from build123d import *

# Parameters (mm, degrees)
SKETCH1_R           = 2
BOSS_EXTRUDE1_DEPTH = 1.4077243
FILLET2_R           = 4


with BuildPart() as part:
    # Sketch1 → Boss-Extrude1 (new body)
    with BuildSketch(Plane(origin=(0, 0, 0), x_dir=(1, 0, 0), z_dir=(0, 1, 0))):
        Polygon((6, -8), (6, 33.34843691), (-61.475760907, 128.370940703), (-81.524239093, 119.312324779), (-104.126855641, 18.58956294), (-104.126855641, -8), align=None)
        with Locations(Location((-96, 0, 0), (0, 0, 270))):
            Circle(SKETCH1_R, mode=Mode.SUBTRACT)
        with Locations(Location((-80, 0, 0), (0, 0, 270))):
            Circle(SKETCH1_R, mode=Mode.SUBTRACT)
        with Locations(Location((-64, 0, 0), (0, 0, 270))):
            Circle(SKETCH1_R, mode=Mode.SUBTRACT)
        with Locations(Location((-97.021679837, 31.983686003, 0), (0, 0, 270))):
            Circle(SKETCH1_R, mode=Mode.SUBTRACT)
        with Locations(Location((-48, 0, 0), (0, 0, 270))):
            Circle(SKETCH1_R, mode=Mode.SUBTRACT)
        with Locations(Location((-32, 0, 0), (0, 0, 270))):
            Circle(SKETCH1_R, mode=Mode.SUBTRACT)
        with Locations(Location((-16, 0, 0), (0, 0, 270))):
            Circle(SKETCH1_R, mode=Mode.SUBTRACT)
        with Locations(Location((0, 0, 0), (0, 0, 270))):
            Circle(SKETCH1_R, mode=Mode.SUBTRACT)
        with Locations(Location((-67.5, 116.913429511, 0), (0, 0, 270))):
            Circle(SKETCH1_R, mode=Mode.SUBTRACT)
    extrude(amount=BOSS_EXTRUDE1_DEPTH)

    # Fillet2
    fillet2_edges = [part.edges().sort_by_distance(p)[0] for p in [
        (6, 0.70386215, 8),
        (-104.126855641, 0.70386215, 8),
        (-104.126855641, 0.70386215, -18.58956294),
        (-81.524239093, 0.70386215, -119.312324779),
        (-61.475760907, 0.70386215, -128.370940703),
        (6, 0.70386215, -33.34843691),
    ]]
    fillet(fillet2_edges, radius=FILLET2_R)


solid = part.part
Check sheet for the modelled part. Datum: model origin and axes. Units: mm. Give positions to 0.01 mm unless a question says otherwise; leave off trailing zeros. Loops run counter-clockwise (first coordinate to the right, second up) from the corner with the lowest first, then second, coordinate; pieces in that order, holes last. Notation, with made-up numbers: M 80.25,13.5 L 125.25,13.5 A11 cw 125.25,32.5 Z; hole C 36,71 d10. An arc over 180 degrees is marked long. Return JSON: item names as keys, results as strings. Group by question number.
1. Mould release check, pull along Z, two halves, no side actions. Record for faces 1 (the flat face through (-71.985, 0.694, -123.623)), 2 (the cylindrical face through (-2, 1, 0)), 3 (the flat face through (-50, 0, -46)), 4 (the cylindrical face through (-102.924, 0.714, 6.859)): released by +Z, released by -Z, zero draft, split by the parting line, or undercut.
2. Cross-section at A-A on z = 0. State how many separate pieces and enclosed holes the cut face has, plus the area to 3 significant figures.
3. Thickness scan on L1, parallel to X at y = 0.5, z = -32.5; L2, parallel to Z at x = -48.5, y = 0.55; L3, parallel to X at y = 0.85, z = -53.5. Record the ranges inside material, lowest first.
4. Cross-section at B-B on x = -48. Record the boundary of the cut face in (y, z), plus the area to 3 significant figures.
5. Go/stop test with a flat-tipped pin: pin 1 (2.5 mm diameter, centred on x = -80, z = 0, fed in from +Y). Record where the tip stops, or that it passes through.
6. Cross-section at D-D on x = -16. Record the boundary of the cut face in (y, z), plus the area to 3 significant figures.
Return value:
{
 "1": {"face 1": "released by -Z", "face 2": "undercut", "face 3": "zero draft", "face 4": "released by +Z"},
 "2": {"separate pieces": "8", "enclosed holes": "0", "area": "116 mm^2"},
 "3": {"L1": "-101.01 to -98.95, -95.09 to 5.98", "L2": "-110.1 to -1.94, 1.94 to 8", "L3": "-96.29 to -8.31"},
 "4": {"outline": "M 0,-109.39 L 1.41,-109.39 L 1.41,-2 L 0,-2 Z; M 0,2 L 1.41,2 L 1.41,8 L 0,8 Z", "area": "160 mm^2"},
 "5": {"pin 1": "through"},
 "6": {"outline": "M 0,-64.33 L 1.41,-64.33 L 1.41,-2 L 0,-2 Z; M 0,2 L 1.41,2 L 1.41,8 L 0,8 Z", "area": "96.2 mm^2"}
}
